The model under review builds one solid part; all positions refer to its coordinate system, in mm. A direction names the side the tool comes from. Coordinates: 2 decimals unless noted, no trailing zeros. Write each loop counter-clockwise with the first axis right and the second up, starting at its lowest first coordinate (ties: lowest second). Pieces come first, ordered by that corner, then holes. Notation, with made-up numbers: (79.25, 85) -> (89.25, 85) arc R5 cw to (89.25, 89) -> close; hole circle Ø2 at (-6.5, 13). An arc over 180 degrees is marked (long way). Write each question's results on one line, items separated by ' | '.
```python
from build123d import *

# Parameters (mm, degrees)
SKETCH1_W                 = 20.32
SKETCH1_H                 = 157.48
BOSS_EXTRUDE1_DEPTH       = 56.896
CHAMFER1_SIZE             = 8.89
SHELL1_T                  = -1.27
F_2_CLEARANCE_HOLE1_D     = 2.4384
F_2_CLEARANCE_HOLE1_DEPTH = 7.62
F_2_CLEARANCE_HOLE1_TIP   = 0.732569267


with BuildPart() as part:
    # Sketch1 → Boss-Extrude1 (new body)
    with BuildSketch(Plane(origin=(0, 0, 0), x_dir=(1, 0, 0), z_dir=(0, 1, 0))):
        with Locations((10.16, 78.74)):
            Rectangle(SKETCH1_W, SKETCH1_H)
    extrude(amount=BOSS_EXTRUDE1_DEPTH)

    # Chamfer1
    chamfer1_edges = [part.edges().sort_by_distance(p)[0] for p in [
        (20.32, 56.896, -78.74),
        (20.32, 0, -78.74),
    ]]
    chamfer(chamfer1_edges, length=CHAMFER1_SIZE)

    # Shell1
    shell1_openings = [part.faces().sort_by_distance(p)[0] for p in [
        (0, 28.448, -78.74),
    ]]
    offset(amount=SHELL1_T, openings=shell1_openings, kind=Kind.INTERSECTION)

    # #2 Clearance Hole1
    with Locations(Plane(origin=(20.32, 0, 0), x_dir=(0, 0, -1), z_dir=(1, 0, 0))):
        with Locations((55.88, 28.448), (72.39, 28.448), (80.645, 36.703), (80.645, 20.193), (88.9, 28.448), (105.41, 28.448), (97.155, 36.703), (97.155, 20.193), (64.135, 36.703), (64.135, 20.193)):
            Hole(F_2_CLEARANCE_HOLE1_D / 2, depth=F_2_CLEARANCE_HOLE1_DEPTH)
            with Locations((0, 0, -(F_2_CLEARANCE_HOLE1_DEPTH + F_2_CLEARANCE_HOLE1_TIP / 2))):  # 118° drill point
                Cone(0, F_2_CLEARANCE_HOLE1_D / 2, F_2_CLEARANCE_HOLE1_TIP, mode=Mode.SUBTRACT)


solid = part.part
```
Q1. Clearance check with a flat-ended pin moving along its axis: P1, Ø4, axis at y = 28.448, z = -72.39, coming from the -X side. State where the tip first meets the part, or that it passes through.
Solution:
P1: x = 19.05
Q2. Add section B-B (z = -100). Write out the cut boundary in (x, y), plus the area to 3 significant figures.
Solution:
outline: (0, 0) -> (11.43, 0) -> (20.32, 8.89) -> (20.32, 48.01) -> (11.43, 56.9) -> (0, 56.9) -> (0, 55.63) -> (10.9, 55.63) -> (19.05, 47.48) -> (19.05, 9.42) -> (10.9, 1.27) -> (0, 1.27) -> close | area: 108 mm²
Q3. Add section C-C (y = 44.5). Write out the cut boundary in (x, z), plus the area to 3 significant figures.
Solution:
outline: (0, -157.48) -> (20.32, -157.48) -> (20.32, 0) -> (0, 0) -> (0, -1.27) -> (19.05, -1.27) -> (19.05, -156.21) -> (0, -156.21) -> close | area: 248 mm²
Q4. Machinability: for faces 4 (the flat face through (15.81, 4.38, -77.64)), 5 (the flat face through (9, 28, -1.27)), which of the approach directions +Z, -Z, +X, -X, +Y, -Y give a long, thin tool a straight path to every point of the face, cutting with its end or side? Answer none if there is none.
Solution:
face 4: +Z, -Z, +X, -Y | face 5: -X
Q5. Add section A-A (x = 2.5). Write out the cut boundary in (y, z).
Solution:
outline: (0, -157.48) -> (56.9, -157.48) -> (56.9, 0) -> (0, 0) -> close; hole (1.27, -156.21) -> (55.63, -156.21) -> (55.63, -1.27) -> (1.27, -1.27) -> close
Q6. Draft analysis for pull direction Z (two halves, no side actions). For faces 1 (the flat face through (5, 55.626, -80)), 2 (the flat face through (10, 28, -157.48)), 3 (the flat face through (6, 0, -80)), state which applies: pulls with the +Z half, pulls with the -Z half, needs draft (parallel to the pull), parting line crosses it, or undercut.
Solution:
face 1: undercut | face 2: pulls with the -Z half | face 3: needs draft
Q7. For line 1 (Z direction, x = 9.5, y = 8); line 2 (Y direction, x = 2.5, z = -60.5); line 3 (X direction, y = 41.5, z = -145), list the stretches that pass through material, from the lowest coordinate up. Write a range as from..to.
Solution:
line 1: -157.48..-156.21, -1.27..0 | line 2: 0..1.27, 55.63..56.9 | line 3: 19.05..20.32
Q8. Add section D-D (x = 14.75). Write out the cut boundary in (y, z).
Solution:
outline: (3.32, -157.48) -> (53.58, -157.48) -> (53.58, 0) -> (3.32, 0) -> close; hole (5.12, -156.21) -> (51.78, -156.21) -> (51.78, -1.27) -> (5.12, -1.27) -> close
